from build123d import *

# Parameters (mm, degrees)
F0_W     = 108.723074
F0_H     = 79.27715
F0_W_2   = 92.569218
F0_H_2   = 63.744598
F1_DEPTH = 70.866
F2_R     = 8.945792
F3_DEPTH = 254
F5_DEPTH = 254


with BuildPart() as f1:
    # F0 (on Top) → F1 (new body)
    with BuildSketch(Plane.XY):
        Rectangle(F0_W, F0_H)
        Rectangle(F0_W_2, F0_H_2, mode=Mode.SUBTRACT)
    extrude(amount=F1_DEPTH)

    # F2 (on face) → F3 (cut)
    with BuildSketch(Plane.YZ.offset(54.361537)):
        with Locations((0, 35.433)):
            Circle(F2_R)
    extrude(amount=-F3_DEPTH, mode=Mode.SUBTRACT)

    # F4 (on face) → F5 (cut)
    with BuildSketch(Plane(origin=(0, 39.638575, 0), x_dir=(-1, 0, 0), z_dir=(0, 1, 0))):
        Polygon((30.48, 70.866), (0, 70.866), (-30.48, 70.866), (-30.48, 37.846), (30.48, 37.846), align=None)
    extrude(amount=-F5_DEPTH, mode=Mode.SUBTRACT)


solid = f1.part
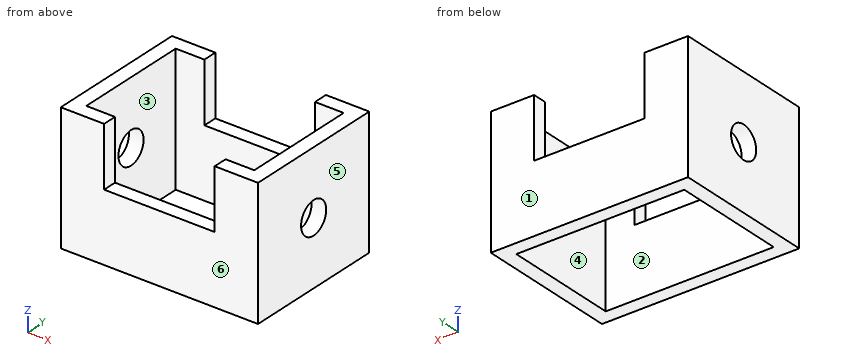
The listing builds one solid part. Answer for the finished solid, in the listing's coordinates (mm). Face numbers are marked on the shaded views. A direction names the side the tool comes from. Round coordinates to 2 decimals unless told otherwise and drop trailing zeros. Write each loop counter-clockwise with the first axis right and the second up, starting at its lowest first coordinate (ties: lowest second). Pieces come first, ordered by that corner, then holes. Notation, with made-up numbers: M 12.5,9.5 L 57.5,9.5 A11 ccw 57.5,18.5 Z; hole C 87.25,26 d7. An arc over 180 degrees is marked long. Write each question's results on one line, items separated by ' | '. Start each with the question number.
(1) The part is cut by section A-A, the plane y = 0. Write down the section's boundary in (x, z), and give its area (3 significant figures).
(2) Each of these flat-tipped pins is pushed along its axis until it touches: P1, Ø21.5, axis at x = -3.5, z = 39.5, coming from the -Y side; P2, Ø4, axis at x = 11.5, y = 36, coming from the +Z side. Where does it stop, or does it pass through?
(3) The part is cut by section B-B, the plane x = 33. Write down the section's boundary in (y, z), and give its area (3 significant figures).
(4) The part is cut by section C-C, the plane z = 47. Write down the section's boundary in (x, y).
(5) The part is cut by section D-D, the plane z = 23. Write down the section's boundary in (x, y), and give its area (3 significant figures).
(6) For the marked faces 1 and 2, determine the directions among +Z, -Z, +X, -X, +Y, -Y from which every point of the face is accessible in a straight line to the end or side of a thin tool.
(7) Find the intervals of material crossed by line 1 (X direction, y = -11.5, z = 7); line 2 (Y direction, x = -22.5, z = 20); line 3 (Z direction, x = 51, y = 0), in increasing order.
(8) Determine the mould class of the marked faces 3, 4, 5 and 6 for opening direction Y: +Y half, -Y half, draft (parallel to the pull), parting line (faces both ways), or undercut.
Worked answers:
1) outline: M -54.36,0 L -46.28,0 L -46.28,26.49 L -54.36,26.49 Z; M -54.36,44.38 L -46.28,44.38 L -46.28,70.87 L -54.36,70.87 Z; M 46.28,0 L 54.36,0 L 54.36,26.49 L 46.28,26.49 Z; M 46.28,44.38 L 54.36,44.38 L 54.36,70.87 L 46.28,70.87 Z | area: 856 mm²
2) P1: stops at y = -39.64 | P2: stops at z = 37.85
3) outline: M -39.64,0 L -31.87,0 L -31.87,70.87 L -39.64,70.87 Z; M 31.87,0 L 39.64,0 L 39.64,70.87 L 31.87,70.87 Z | area: 1,100 mm²
4) outline: M -54.36,-39.64 L -30.48,-39.64 L -30.48,-31.87 L -46.28,-31.87 L -46.28,31.87 L -30.48,31.87 L -30.48,39.64 L -54.36,39.64 Z; M 30.48,-39.64 L 54.36,-39.64 L 54.36,39.64 L 30.48,39.64 L 30.48,31.87 L 46.28,31.87 L 46.28,-31.87 L 30.48,-31.87 Z
5) outline: M -54.36,-39.64 L 54.36,-39.64 L 54.36,39.64 L -54.36,39.64 Z; hole M -46.28,-31.87 L 46.28,-31.87 L 46.28,31.87 L -46.28,31.87 Z | area: 2,720 mm²
6) face 1: +Z, -Z, +X, -X, +Y | face 2: +Z, -Z
7) line 1: x = -54.36 to -46.28, 46.28 to 54.36 | line 2: y = -39.64 to -31.87, 31.87 to 39.64 | line 3: z = 0 to 26.49, 44.38 to 70.87
8) face 3: undercut | face 4: undercut | face 5: draft | face 6: -Y half
